from build123d import *

# Parameters (mm, degrees)
RUN_HUB_START       = -8
SKETCH1_R           = 6
RUN_HUB_DEPTH       = 16
BRANCH_HUB_START    = -13
SKETCH2_R           = 6
BRANCH_HUB_DEPTH    = 13
BARB_FRONT_START    = 8
SKETCH3_R           = 3
BARB_FRONT_DEPTH    = 12
BARB_BACK_START     = -20
SKETCH4_R           = 3
BARB_BACK_DEPTH     = 12
BARB_BRANCH_START   = -25
SKETCH5_R           = 3
BARB_BRANCH_DEPTH   = 12
RUN_BORE_DEPTH      = 33.57299495
RUN_BORE_DEPTH_BACK = 33.57299495
SKETCH6_R           = 2
BRANCH_BORE_START   = -26
SKETCH7_R           = 2
BRANCH_BORE_DEPTH   = 26


with BuildPart() as part:
    # Sketch1 → Run_Hub (new body)
    with BuildSketch(Plane.XY.offset(RUN_HUB_START)):
        Circle(SKETCH1_R)
    extrude(amount=RUN_HUB_DEPTH)

    # Sketch2 → Branch_Hub (add)
    with BuildSketch(Plane(origin=(0, 0, 0), x_dir=(0, 0, -1), z_dir=(1, 0, 0)).offset(BRANCH_HUB_START)):
        with Locations(Location((0, 0, 0), (0, 0, 270))):
            Circle(SKETCH2_R)
    extrude(amount=BRANCH_HUB_DEPTH)

    # Sketch3 → Barb_Front (add)
    with BuildSketch(Plane.XY.offset(BARB_FRONT_START)):
        Circle(SKETCH3_R)
    extrude(amount=BARB_FRONT_DEPTH)

    # Sketch4 → Barb_Back (add)
    with BuildSketch(Plane.XY.offset(BARB_BACK_START)):
        Circle(SKETCH4_R)
    extrude(amount=BARB_BACK_DEPTH)

    # Sketch5 → Barb_Branch (add)
    with BuildSketch(Plane(origin=(0, 0, 0), x_dir=(0, 0, -1), z_dir=(1, 0, 0)).offset(BARB_BRANCH_START)):
        Circle(SKETCH5_R)
    extrude(amount=BARB_BRANCH_DEPTH)

    # Sketch6 → Run_Bore (cut, two sides: drawn at the far end of the back side and taken through both)
    with BuildSketch(Plane.XY.offset(-RUN_BORE_DEPTH_BACK)):
        Circle(SKETCH6_R)
    extrude(amount=RUN_BORE_DEPTH + RUN_BORE_DEPTH_BACK, mode=Mode.SUBTRACT)

    # Sketch7 → Branch_Bore (cut)
    with BuildSketch(Plane(origin=(0, 0, 0), x_dir=(0, 0, -1), z_dir=(1, 0, 0)).offset(BRANCH_BORE_START)):
        with Locations(Location((0, 0, 0), (0, 0, 90))):
            Circle(SKETCH7_R)
    extrude(amount=BRANCH_BORE_DEPTH, mode=Mode.SUBTRACT)


solid = part.part
Build history of the part. All positions in model axes, mm. A direction names the side the tool comes from. Round coordinates to 2 decimals unless told otherwise and drop trailing zeros. Write each loop counter-clockwise with the first axis right and the second up, starting at its lowest first coordinate (ties: lowest second). Pieces come first, ordered by that corner, then holes. Notation, with made-up numbers: (-6.75, -39) -> (25.25, -39) arc R31 cw to (25.25, -14) -> close; hole circle Ø3 at (-1.75, -33). An arc over 180 degrees is marked (long way). Write item = value, one per line.
(1) Band-saw the part on B-B (x = -1.5). Give the cut face in (y, z), then the cut area to 3 significant figures.
Answer:
outline = (-5.81, -8) -> (-2.6, -8) -> (-2.6, -20) -> (-1.32, -20) -> (-1.32, -1.5) arc R2 cw to (-1.32, 1.5) -> (-1.32, 20) -> (-2.6, 20) -> (-2.6, 8) -> (-5.81, 8) -> (-5.81, 1.5) arc R6 ccw to (-5.81, -1.5) -> close; (1.32, -20) -> (2.6, -20) -> (2.6, -8) -> (5.81, -8) -> (5.81, -1.5) arc R6 ccw to (5.81, 1.5) -> (5.81, 8) -> (2.6, 8) -> (2.6, 20) -> (1.32, 20) -> (1.32, 1.5) arc R2 cw to (1.32, -1.5) -> close
area = 203 mm2
(2) Band-saw the part on C-C (z = 0). Give the cut face in (x, y), then the cut area to 3 significant figures.
Answer:
outline = (-25, -3) -> (-13, -3) -> (-13, -6) -> (0, -6) arc R6 ccw to (0, 6) -> (-13, 6) -> (-13, 3) -> (-25, 3) -> (-25, 2) -> (0, 2) arc R2 cw to (0, -2) -> (-25, -2) -> close
area = 178 mm2
(3) Tool access for faces 1 (the face through (1.908, 0.601, -0.28)), 2 (the face through (-3, 0, 14)), 3 (the face through (-3, 0, -14)), 4 (the face through (5.723, 1.802, -0.112)), 5 (the face through (-19, 0, 3)): list every direction of +Z, -Z, +X, -X, +Y, -Y with a clear straight run to the whole face (end or side of a thin tool).
Answer:
face_1 = +Z, -Z
face_2 = +Z
face_3 = -Z
face_4 = none
face_5 = -X
(4) Band-saw the part on D-D (y = -4.75). Give the cut face in (x, z), then the cut area to 3 significant figures.
Answer:
outline = (-13, -3.67) -> (-3.67, -3.67) -> (-3.67, -8) -> (3.67, -8) -> (3.67, 8) -> (-3.67, 8) -> (-3.67, 3.67) -> (-13, 3.67) -> close
area = 186 mm2
(5) Probe L1, parallel to Z at x = -7.25, y = 0; L2, parallel to Y at x = 0, z = 10. List the from-to ranges inside material, lowest first.
Answer:
L1 = -6 to -2, 2 to 6
L2 = -3 to -2, 2 to 3
(6) Two-plate mould, pull along Z, no slides. Class faces 6 (the face through (-8.04, 4.42, -4.06)), 7 (the face through (-13, -2, 0)), 8 (the face through (-3, -1, -8)): pulls with the +Z half, pulls with the -Z half, needs draft (parallel to the pull), parting line crosses it, or undercut.
Answer:
face_6 = parting line crosses it
face_7 = undercut
face_8 = pulls with the -Z half
(7) Flat gauge pins, fed straight in: pin 1 (2 mm diameter, centred on x = -5.5, y = -2.5, fed in from +Z); pin 2 (6 mm diameter, centred on x = -9, y = 2.5, fed in from +Z); pin 3 (2 mm diameter, centred on y = -0.5, z = -15.5, fed in from +X); pin 4 (2.5 mm diameter, centred on x = 0, y = 0, fed in from -Z). Where does each tip first touch, or does it go through?
Answer:
pin_1 = 8
pin_2 = 6
pin_3 = 3
pin_4 = through
(8) Band-saw the part on A-A (y = 0). Give the cut face in (x, z).
Answer:
outline = (-25, -3) -> (-13, -3) -> (-13, -6) -> (-6, -6) -> (-6, -8) -> (-3, -8) -> (-3, -20) -> (-2, -20) -> (-2, -2) -> (-25, -2) -> close; (-25, 2) -> (-2, 2) -> (-2, 20) -> (-3, 20) -> (-3, 8) -> (-6, 8) -> (-6, 6) -> (-13, 6) -> (-13, 3) -> (-25, 3) -> close; (2, -20) -> (3, -20) -> (3, -8) -> (6, -8) -> (6, 8) -> (3, 8) -> (3, 20) -> (2, 20) -> close
